Geometry check sheet. Reference: the model listing, model coordinates, mm. Give positions to 0.01 mm unless a question says otherwise; leave off trailing zeros. Loops run counter-clockwise (first coordinate to the right, second up) from the corner with the lowest first, then second, coordinate; pieces in that order, holes last.
1. Material ranges on L1, parallel to Z at x = -6.25, y = -0.7; L2, parallel to X at y = -0.4, z = -12; L3, parallel to X at y = -0.4, z = 16, recorded low to high.
2. Cross-section at C-C, the plane y = -0.4. Record the cut outline in (x, z), plus the area to 3 significant figures.
3. Cross-section at B-B, the plane x = 14.25. Record the cut outline in (y, z).
4. Go/stop test with a flat-tipped pin: pin 1 Ø0.8 at (y, z) = (-1, 15.5) entering from +X. Record where the tip stops, or that it passes through.
from build123d import *

# Parameters (mm, degrees)
F0_W     = 4
F0_H     = 25
F1_DEPTH = 1.5
F2_R     = 0.74999
F3_SIZE  = 0.7


# Not quite as in the source:
# - a fillet or chamfer is up to 0.001 mm smaller than in the source, because OpenCascade refuses the exact size


with BuildPart() as f1:
    # F0 (on Front) → F1 (new body)
    with BuildSketch(Plane.XZ):
        Polygon((-9.8700001836, 17.5), (-12, 17.5), (-12, -17.5), (-9.8700001836, -17.5), (-9.8700001836, -12.5), (10.1299998164, -12.5), (10.1299998164, -17.5), (12, -17.5), (12, -12.1500007808), (12, 12.8499992192), (12, 17.5), (10.1299998164, 17.5), (10.1299998164, 12.5), (-9.8700001836, 12.5), align=None)
        with Locations((14, 0.3499992192)):
            Rectangle(F0_W, F0_H)
    extrude(amount=F1_DEPTH)

    # F2 (radius 0.75 in the source; OpenCascade refuses exactly that, so slightly less here)
    f2_edges = [f1.edges().sort_by_distance(p)[0] for p in [
        (0.13, -1.5, 12.5),
        (0.13, -1.5, -12.5),
        (0.13, 0, -12.5),
        (0.13, 0, 12.5),
        (10.13, 0, 15),
        (-9.87, 0, 15),
        (-9.87, -1.5, 15),
        (-9.87, -1.5, -15),
        (-9.87, 0, -15),
        (10.13, -1.5, -15),
        (10.13, 0, -15),
        (10.13, -1.5, 15),
    ]]
    fillet(f2_edges, radius=F2_R)

    # F3
    f3_edges = [f1.edges().sort_by_distance(p)[0] for p in [
        (16, -1.5, 0.349999),
        (16, 0, 0.349999),
        (14, -1.5, -12.150001),
        (14, 0, -12.150001),
        (14, 0, 12.849999),
        (14, -1.5, 12.849999),
    ]]
    chamfer(f3_edges, length=F3_SIZE)


solid = f1.part
Result:
1. L1: z = -12.5 to 12.5
1. L2: x = -12 to 12
1. L3: x = -12 to -9.96, 10.22 to 12
2. outline: (-12, -17.5) - (-9.96, -17.5) - (-9.96, -12.41) - (10.22, -12.41) - (10.22, -17.5) - (12, -17.5) - (12, -11.85) - (15.7, -11.85) - (15.7, 12.55) - (12, 12.55) - (12, 17.5) - (10.22, 17.5) - (10.22, 12.41) - (-9.96, 12.41) - (-9.96, 17.5) - (-12, 17.5) - close
2. area: 725 mm2
3. outline: (-1.5, -11.45) - (-0.8, -12.15) - (-0.7, -12.15) - (0, -11.45) - (0, 12.15) - (-0.7, 12.85) - (-0.8, 12.85) - (-1.5, 12.15) - close
4. pin 1: stops at x = 12
